For this review, take the finished solid that the model builds, in its own axes (mm). Face numbers are marked on the shaded views. A direction names the side the tool comes from. Give positions to 0.01 mm unless a question says otherwise; leave off trailing zeros. Write each loop counter-clockwise with the first axis right and the second up, starting at its lowest first coordinate (ties: lowest second). Pieces come first, ordered by that corner, then holes. Notation, with made-up numbers: M -35,-32 L 16,-32 A38 cw 16,6 Z; hole C 53,-21 d10. An arc over 180 degrees is marked long. Write item = value, one per line.
```python
from build123d import *

# Parameters (mm, degrees)
F0_W          = 139.7
F0_H          = 55.88
F1_DEPTH      = 55.88
F2_R          = 27.93999
F3_W          = 53.34
F3_H          = 25.4
F4_DEPTH      = 6.9680017111
F4_DEPTH_BACK = 48.9139982889


# Not quite as in the source:
# - a fillet or chamfer is up to 0.001 mm smaller than in the source, because OpenCascade refuses the exact size


with BuildPart() as f1:
    # F0 (on Top) → F1 (new body)
    with BuildSketch(Plane.XY):
        with Locations((19.5538900733, -20.9729982889)):
            Rectangle(F0_W, F0_H)
    extrude(amount=F1_DEPTH)

    # F2 (radius 27.94 in the source; OpenCascade refuses exactly that, so slightly less here)
    f2_edges = [f1.edges().sort_by_distance(p)[0] for p in [
        (-50.29611, -20.972998, 0),
        (-50.29611, -20.972998, 55.88),
        (89.40389, -48.912998, 27.94),
        (89.40389, 6.967002, 27.94),
    ]]
    fillet(f2_edges, radius=F2_R)

    # F3 (on Front) → F4 (cut, two sides)
    with BuildSketch(Plane.XZ) as f4_sk:
        with Locations((62.7338900733, 27.94)):
            Rectangle(F3_W, F3_H)
    extrude(amount=-F4_DEPTH, mode=Mode.SUBTRACT)
    extrude(f4_sk.sketch, amount=F4_DEPTH_BACK, mode=Mode.SUBTRACT)


solid = f1.part
```
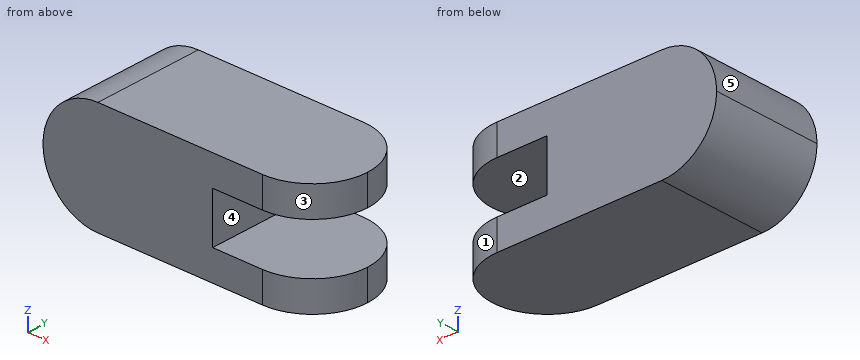
1. Insertion check: P1, Ø3, axis at y = -1.5, z = 42, coming from the +X side; P2, Ø12, axis at y = -25.5, z = 43, coming from the -X side. Each pin has a flat end and moves straight along its axis. Give the tip position at first contact, or say it passes through.
Responses:
P1 = 82.86
P2 = -48.79
2. For line 1 along Z through (x, y) = (68, -5.5); line 2 along X through (y, z) = (-39, 50.5); line 3 along X through (y, z) = (-34.5, 8.5), list the stretches that pass through material, from the lowest coordinate up. Write a range as from..to.
Responses:
line_1 = 0..15.24, 40.64..55.88
line_2 = -38.84..82.81
line_3 = -42.42..85.91
3. Machinability: for the marked faces 1 and 2, which of the approach directions +Z, -Z, +X, -X, +Y, -Y give a long, thin tool a straight path to every point of the face, cutting with its end or side? Answer none if there is none.
Responses:
face_1 = +Z, -Z, +X, +Y
face_2 = +X, +Y, -Y
4. We need section D-D, the plane x = -31. Write out the cut boundary in (y, z).
Responses:
outline = M -48.91,1.37 L 6.97,1.37 L 6.97,54.51 L -48.91,54.51 Z
5. We need section A-A, the plane x = 46. Write out the cut boundary in (y, z).
Responses:
outline = M -48.91,0 L 6.97,0 L 6.97,15.24 L -48.91,15.24 Z; M -48.91,40.64 L 6.97,40.64 L 6.97,55.88 L -48.91,55.88 Z
6. The part is to be moulded in two halves that separate along Z. For the marked faces 3, 4 and 5, say which applies: +Z half, -Z half, draft (parallel to the pull), parting line (faces both ways), or undercut.
Responses:
face_3 = draft
face_4 = undercut
face_5 = +Z half
